Can you work these out from the drawing? Everything is in mm from the part's minimum corner. A direction names the side the tool comes from. Coordinates: 2 decimals unless noted, no trailing zeros. Order: outer loops, then holes, each group sorted by start corner. A loop starts at its lowest first (then second) coordinate and runs counter-clockwise, first axis right, second up. Notation, with made-up numbers: (89, -5) - (122, -5) arc R32 cw to (122, 26) - close; hole circle Ø10 at (10.5, -13.5). An arc over 180 degrees is marked (long way). Answer as CSV lines item,"result". Start each with the question number.
Q1. Suppose I cut it at D-D (z = 9.25). Please give me the cut outline in (x, y).
Q2. Suppose I cut it at B-B (x = 2.75). Please give me the cut outline in (y, z).
Q3. For the marked faces 1, 2 and 3, which set-ups out of +Z, -Z, +X, -X, +Y, -Y let a thin tool reach every point of the face, with its end or its side?
Q4. I need wall thicknesses on line 1 (X direction, y = 1, z = 10.25); line 2 (Y direction, x = 2, z = 11); line 3 (Z direction, x = 2.5, y = 4.1). Which ranges of each line are inside material? Lowest first, please.
Q5. Suppose I cut it at C-C (y = 1.3). Please give me the cut outline in (x, z).
Q6. Suppose I cut it at A-A (y = 3.45). Please give me the cut outline in (x, z), then the cut area to 3 significant figures.
Q7. For pin 1 Ø1.5 at (y, z) = (2.5, 12) entering from +X; pin 2 Ø9.5 at (x, z) = (5, 4) entering from +Y; pin 3 Ø0.9 at (y, z) = (4, 2.5) entering from -X, each with a flat end and sliding along its axis, tell me the tip position at first contact or that it passes through.
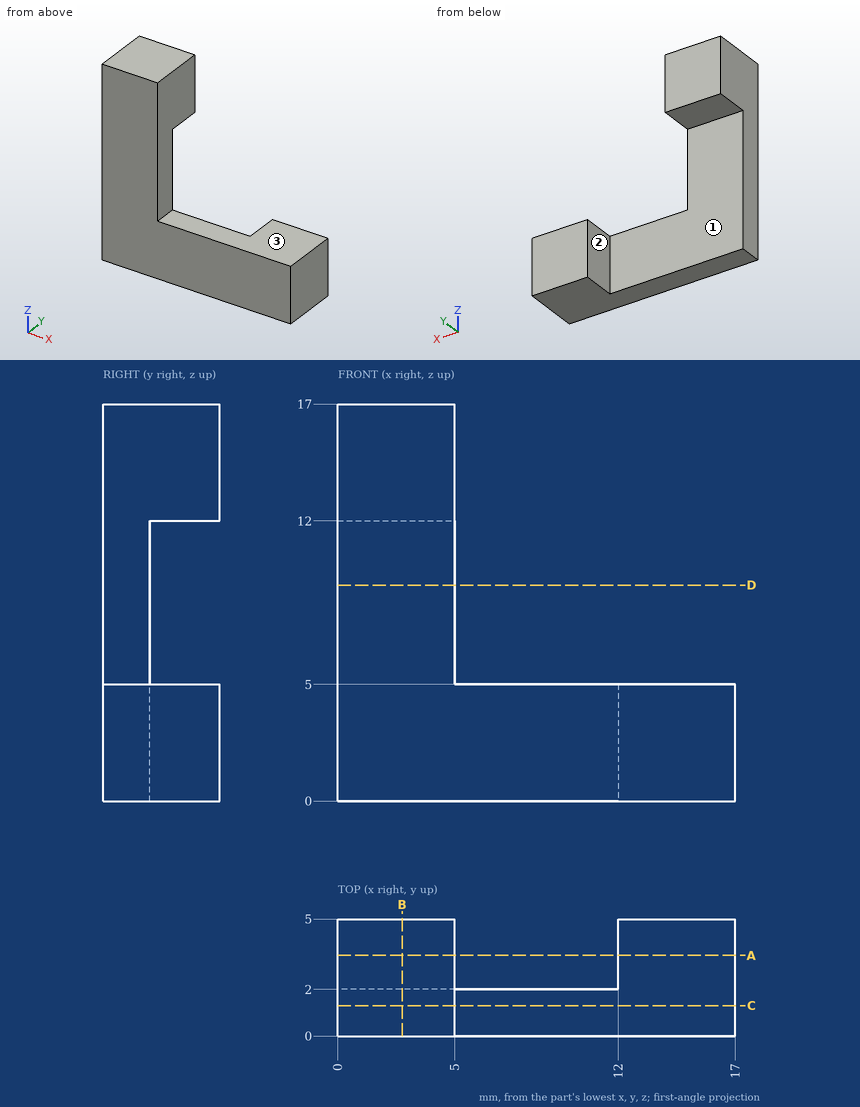
Here are the results:
1,outline,"(0, 0) - (5, 0) - (5, 2) - (0, 2) - close"
2,outline,"(0, 0) - (2, 0) - (2, 12) - (5, 12) - (5, 17) - (0, 17) - close"
3,face 1,"-Z, -X, +Y"
3,face 2,"+Z, -Z, -X, +Y"
3,face 3,"+Z, +X, +Y, -Y"
4,line 1,"x = 0 to 5"
4,line 2,"y = 0 to 2"
4,line 3,"z = 12 to 17"
5,outline,"(0, 0) - (17, 0) - (17, 5) - (5, 5) - (5, 17) - (0, 17) - close"
6,outline,"(0, 12) - (5, 12) - (5, 17) - (0, 17) - close; (12, 0) - (17, 0) - (17, 5) - (12, 5) - close"
6,area,"50.0 mm²"
7,pin 1,"stops at x = 5"
7,pin 2,"stops at y = 2"
7,pin 3,"stops at x = 12"
